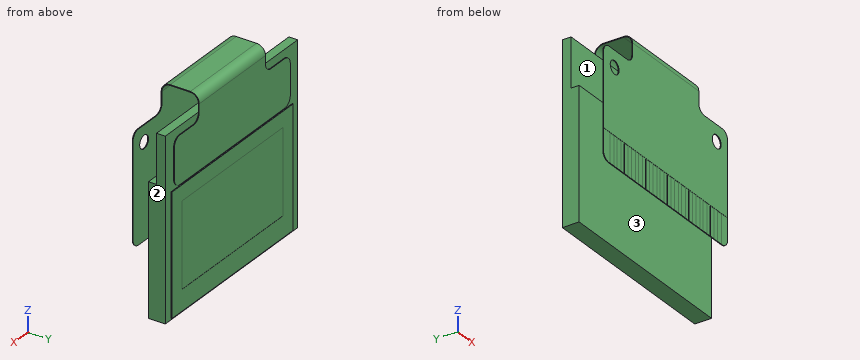
from build123d import *

# Parameters (mm, degrees)
SKETCH1_W           = 12
SKETCH1_H           = 11
BOSS_EXTRUDE1_DEPTH = 1.1
SKETCH2_W           = 12
SKETCH2_H           = 11
SKETCH2_W_2         = 11
SKETCH2_H_2         = 7.4
CUT_EXTRUDE1_DEPTH  = 0.06
SKETCH3_W           = 9.196
SKETCH3_H           = 5.18
CUT_EXTRUDE2_DEPTH  = 0.01
SKETCH4_W           = 12
SKETCH4_H           = 3
CUT_EXTRUDE3_DEPTH  = 0.5
BOSS_EXTRUDE2_DEPTH = 0.05
BOSS_EXTRUDE3_DEPTH = 3
SKETCH7_W           = 11.25
SKETCH7_H           = 6.8
SKETCH7_R           = 0.4
BOSS_EXTRUDE4_DEPTH = 0.05
SKETCH8_W           = 0.3
SKETCH8_H           = 1.8
SKETCH8_W_2         = 0.575
CUT_EXTRUDE4_DEPTH  = 0.01
SKETCH10_W          = 10.1
SKETCH10_H          = 0.05
CUT_EXTRUDE5_DEPTH  = 0.01
FILLET1_R           = 0.5


with BuildPart() as part:
    # Sketch1 → Boss-Extrude1 (new body)
    with BuildSketch(Plane(origin=(0, 0, 0), x_dir=(1, 0, 0), z_dir=(0, 1, 0))):
        Rectangle(SKETCH1_W, SKETCH1_H)
    extrude(amount=BOSS_EXTRUDE1_DEPTH)

    # Sketch2 → Cut-Extrude1 (cut)
    with BuildSketch(Plane(origin=(0, 1.1, 0), x_dir=(1, 0, 0), z_dir=(0, 1, 0))):
        Rectangle(SKETCH2_W, SKETCH2_H)
        with Locations((0, 1.7)):
            Rectangle(SKETCH2_W_2, SKETCH2_H_2, mode=Mode.SUBTRACT)
    extrude(amount=-CUT_EXTRUDE1_DEPTH, mode=Mode.SUBTRACT)

    # Sketch3 → Cut-Extrude2 (cut)
    with BuildSketch(Plane(origin=(0, 1.1, 0), x_dir=(1, 0, 0), z_dir=(0, 1, 0))):
        with Locations((0, 1.535)):
            Rectangle(SKETCH3_W, SKETCH3_H)
    extrude(amount=-CUT_EXTRUDE2_DEPTH, mode=Mode.SUBTRACT)

    # Sketch4 → Cut-Extrude3 (cut)
    with BuildSketch(Plane.XZ):
        with Locations((0, 4)):
            Rectangle(SKETCH4_W, SKETCH4_H)
    extrude(amount=-CUT_EXTRUDE3_DEPTH, mode=Mode.SUBTRACT)

    # Sketch5 → Boss-Extrude2 (add)
    with BuildSketch(Plane(origin=(0, 1.04, 0), x_dir=(1, 0, 0), z_dir=(0, 1, 0))):
        with BuildLine():
            Line((-4.75, -2.1), (4.75, -2.1))
            ThreePointArc((4.75, -2.1), (5.103553391, -2.246446609), (5.25, -2.6))
            Line((5.25, -2.6), (5.25, -4.5))
            ThreePointArc((5.25, -4.5), (5.103553391, -4.853553391), (4.75, -5))
            Line((4.75, -5), (3.5, -5))
            ThreePointArc((3.5, -5), (3.146446609, -5.146446609), (3, -5.5))
            Line((3, -5.5), (3, -6))
            Line((3, -6), (-3, -6))
            Line((-3, -6), (-3, -5.5))
            ThreePointArc((-3, -5.5), (-3.146446609, -5.146446609), (-3.5, -5))
            Line((-3.5, -5), (-4.75, -5))
            ThreePointArc((-4.75, -5), (-5.103553391, -4.853553391), (-5.25, -4.5))
            Line((-5.25, -4.5), (-5.25, -2.6))
            ThreePointArc((-5.25, -2.6), (-5.103553391, -2.246446609), (-4.75, -2.1))
        make_face()
    extrude(amount=BOSS_EXTRUDE2_DEPTH)

    # Sketch6 → Boss-Extrude3 (add, symmetric)
    with BuildSketch(Plane(origin=(0, 0, 0), x_dir=(0, 0, -1), z_dir=(1, 0, 0))):
        with BuildLine():
            Line((-6.5, 0.54), (-6.5, -0.7))
            ThreePointArc((-6.5, -0.7), (-6.353553391, -1.053553391), (-6, -1.2))
            Line((-6, -1.2), (2, -1.2))
            Line((2, -1.2), (2, -1.25))
            Line((2, -1.25), (-6, -1.25))
            ThreePointArc((-6, -1.25), (-6.38890873, -1.08890873), (-6.55, -0.7))
            Line((-6.55, -0.7), (-6.55, 0.54))
            ThreePointArc((-6.55, 0.54), (-6.38890873, 0.92890873), (-6, 1.09))
            Line((-6, 1.09), (-6, 1.04))
            ThreePointArc((-6, 1.04), (-6.353553391, 0.893553391), (-6.5, 0.54))
        make_face()
    extrude(amount=BOSS_EXTRUDE3_DEPTH, both=True)

    # Sketch7 → Boss-Extrude4 (add)
    with BuildSketch(Plane.XZ.offset(1.25)):
        with Locations((0, 1.4)):
            Rectangle(SKETCH7_W, SKETCH7_H)
        with Locations((-4.625, 3.8)):
            Circle(SKETCH7_R, mode=Mode.SUBTRACT)
        with Locations((4.625, 3.8)):
            Circle(SKETCH7_R, mode=Mode.SUBTRACT)
    extrude(amount=-BOSS_EXTRUDE4_DEPTH)

    # Sketch8 → Cut-Extrude4 (cut)
    with BuildSketch(Plane.XZ.offset(1.25)):
        with Locations((0, -1.1)):
            Rectangle(SKETCH8_W, SKETCH8_H)
        with Locations((0.65, -1.1)):
            Rectangle(SKETCH8_W, SKETCH8_H)
        with Locations((1.3, -1.1)):
            Rectangle(SKETCH8_W, SKETCH8_H)
        with Locations((1.95, -1.1)):
            Rectangle(SKETCH8_W, SKETCH8_H)
        with Locations((2.6, -1.1)):
            Rectangle(SKETCH8_W, SKETCH8_H)
        with Locations((3.25, -1.1)):
            Rectangle(SKETCH8_W, SKETCH8_H)
        with Locations((3.9, -1.1)):
            Rectangle(SKETCH8_W, SKETCH8_H)
        with Locations((4.55, -1.1)):
            Rectangle(SKETCH8_W, SKETCH8_H)
        with Locations((-4.55, -1.1)):
            Rectangle(SKETCH8_W, SKETCH8_H)
        with Locations((-3.9, -1.1)):
            Rectangle(SKETCH8_W, SKETCH8_H)
        with Locations((-3.25, -1.1)):
            Rectangle(SKETCH8_W, SKETCH8_H)
        with Locations((-2.6, -1.1)):
            Rectangle(SKETCH8_W, SKETCH8_H)
        with Locations((-1.95, -1.1)):
            Rectangle(SKETCH8_W, SKETCH8_H)
        with Locations((-1.3, -1.1)):
            Rectangle(SKETCH8_W, SKETCH8_H)
        with Locations((-0.65, -1.1)):
            Rectangle(SKETCH8_W, SKETCH8_H)
        with Locations((5.3375, -1.1)):
            Rectangle(SKETCH8_W_2, SKETCH8_H)
        with Locations((-5.3375, -1.1)):
            Rectangle(SKETCH8_W_2, SKETCH8_H)
    extrude(amount=-CUT_EXTRUDE4_DEPTH, mode=Mode.SUBTRACT)

    # Sketch10 → Cut-Extrude5 (cut)
    with BuildSketch(Plane.XZ.offset(1.25)):
        with Locations((0, -0.225)):
            Rectangle(SKETCH10_W, SKETCH10_H)
    extrude(amount=-CUT_EXTRUDE5_DEPTH, mode=Mode.SUBTRACT)

    # Fillet1
    fillet1_edges = [part.edges().sort_by_distance(p)[0] for p in [
        (5.625, -1.22, -2),
        (-5.625, -1.225, 4.8),
        (5.625, -1.225, 4.8),
        (3, -1.225, 4.8),
        (-3, -1.225, 4.8),
        (-5.625, -1.22, -2),
    ]]
    fillet(fillet1_edges, radius=FILLET1_R)


solid = part.part
Verification items for the finished model (mm, model axes). Face numbers are marked on the shaded views. A direction names the side the tool comes from. Give positions to 0.01 mm unless a question says otherwise; leave off trailing zeros. Order: outer loops, then holes, each group sorted by start corner. A loop starts at its lowest first (then second) coordinate and runs counter-clockwise, first axis right, second up. Notation, with made-up numbers: (46, 51) -> (97, 51) arc R29 cw to (97, 80) -> close; hole circle Ø8 at (-1, 20.5). An arc over 180 degrees is marked (long way). Answer as CSV lines item,"result".
Q1. Access from +Z, -Z, +X, -X, +Y, -Y to the whole of each face (thin tool, end or side, straight path). Record for the marked faces 1, 2 and 3.
Solutions:
face 1,"+X, -X"
face 2,"+Z, -Z, +X, +Y, -Y"
face 3,"-Z, +X, -X"
Q2. Sectioned sample at D-D on y = -0.5. Record the cut outline in (x, z).
Solutions:
outline,"(-3, 6.5) -> (3, 6.5) -> (3, 6.55) -> (-3, 6.55) -> close"
Q3. Scan lines: probe 1 along Z at (x, y) = (-4, 0.1); probe 2 along Y at (x, z) = (4.25, -2.75). Record each from-to range of solid material in increasing order.
Solutions:
probe 1,"z = -5.5 to 2.5"
probe 2,"y = 0 to 1.09"
Q4. Sectioned sample at A-A on z = 3.8. Record the cut outline in (x, y) (3 decimals), plus the area to 3 significant figures.
Solutions:
outline,"(-6, 0.5) -> (6, 0.5) -> (6, 1.04) -> (5.25, 1.04) -> (5.25, 1.09) -> (-5.25, 1.09) -> (-5.25, 1.04) -> (-6, 1.04) -> close; (-5.625, -1.25) -> (-5.025, -1.25) -> (-5.025, -1.2) -> (-5.625, -1.2) -> close; (-4.225, -1.25) -> (4.225, -1.25) -> (4.225, -1.2) -> (-4.225, -1.2) -> close; (5.025, -1.25) -> (5.625, -1.25) -> (5.625, -1.2) -> (5.025, -1.2) -> close"
area,"7.49 mm²"
